Part print with two shaded views. Sizes in mm from the minimum x, y, z corner. A direction names the side the tool comes from. Coordinates: 2 decimals unless noted, no trailing zeros. Write each loop counter-clockwise with the first axis right and the second up, starting at its lowest first coordinate (ties: lowest second). Pieces come first, ordered by that corner, then holes. Notation, with made-up numbers: (-40, -13) - (7, -13) arc R23 cw to (7, 9) - close; hole circle Ø9 at (-16.5, 20.25). An arc over 180 degrees is marked (long way). One line per question, with ' | ' between items. Start each with the question number.
1. Band-saw the part on C-C, the plane x = 48.5. Write the cut outline in (y, z).
2. Two-plate mould, pull along Z, no slides. Class the marked faces 6, 7, 8 and 9: +Z half, -Z half, draft (parallel to the pull), parting line (faces both ways), or undercut.
3. Band-saw the part on B-B, the plane z = 55. Write the cut outline in (x, y).
4. Which spindle directions (+Z, -Z, +X, -X, +Y, -Y) get a long thin tool onto all of the face, cutting with end or side? Do the marked faces 1, 2, 3, 4 and 5. Say none if no direction does.
5. Flat gauge pins, fed straight in: P1, Ø15, axis at x = 81.5, y = 31, coming from the +Z side; P2, Ø6, axis at y = 36, z = 51.5, coming from the +X side; P3, Ø4.5, axis at x = 120, y = 32, coming from the +Z side; P4, Ø23, axis at x = 63.5, z = 63.5, coming from the -Y side. Where does each tip first touch, or does it go through?
6. Probe line 1 (Z direction, x = 63.5, y = 39); line 2 (Y direction, x = 63, z = 84); line 3 (Z direction, x = 45, y = 47). List the from-to ranges inside material, lowest first.
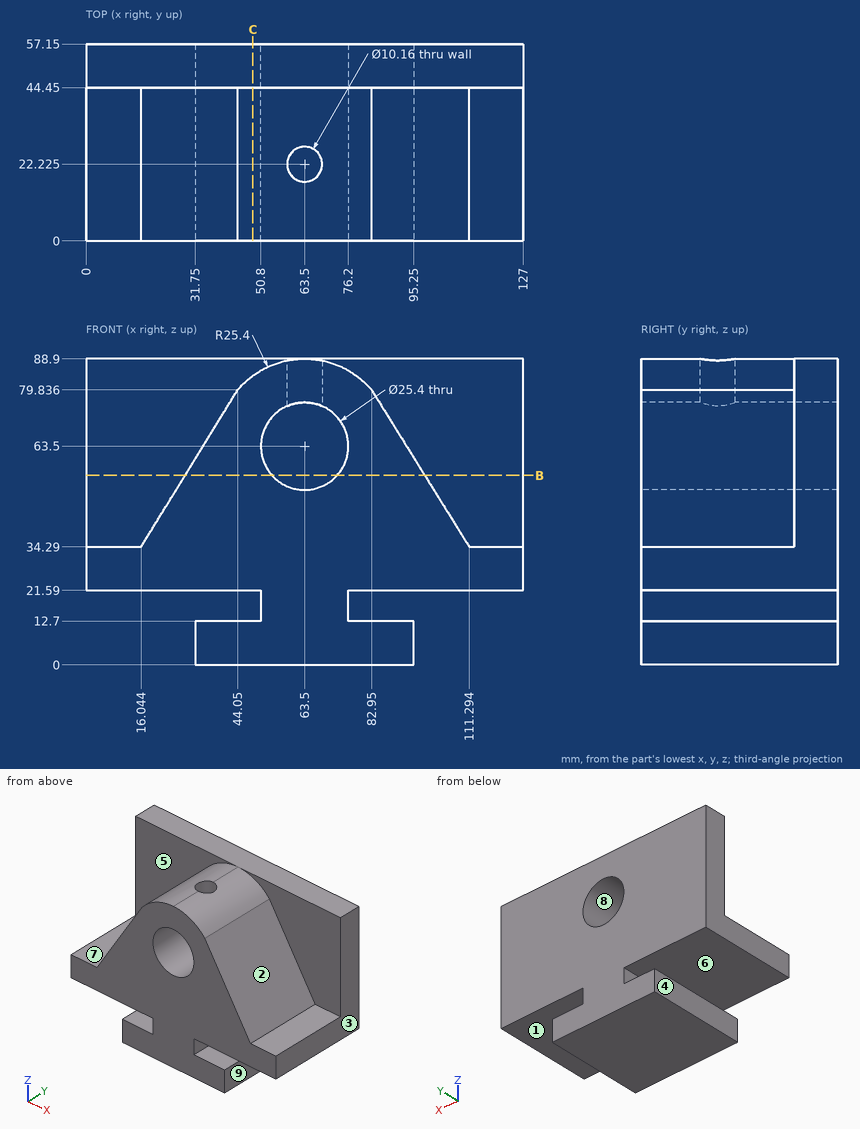
Filled in:
1) outline: (0, 0) - (57.15, 0) - (57.15, 12.7) - (0, 12.7) - close; (0, 21.59) - (57.15, 21.59) - (57.15, 88.9) - (44.45, 88.9) - (44.45, 84) - (0, 84) - close
2) face 6: undercut | face 7: +Z half | face 8: undercut | face 9: draft
3) outline: (0, 44.45) - (28.78, 44.45) - (28.78, 0) - (54.06, 0) - (54.06, 57.15) - (0, 57.15) - close; (72.94, 0) - (98.41, 0) - (98.41, 44.45) - (127, 44.45) - (127, 57.15) - (72.94, 57.15) - close
4) face 1: +X, +Y, -Y | face 2: +Z, +X, -Y | face 3: +Z, -Z, +X, +Y, -Y | face 4: -Z, -X, +Y, -Y | face 5: +Z, -X, -Y
5) P1: stops at z = 86.63 | P2: stops at x = 102.45 | P3: stops at z = 34.29 | P4: passes through
6) line 1: z = 0 to 50.8, 76.2 to 88.9 | line 2: y = 0 to 17.17, 27.28 to 57.15 | line 3: z = 0 to 12.7, 21.59 to 88.9
